from build123d import *

# Parameters (mm, degrees)
F0_W        = 76.2
F0_H        = 50.8
F2_DEPTH    = 25.4
F1_W        = 76.2
F1_H        = 8.89
F3_DEPTH    = 8.89
F4_R        = 2.54
F6_DEPTH    = 16.51
F7_R        = 5.08
F8_T        = 2.54
F8_T3_DEPTH = 10.16
F8_T5_DEPTH = 37.1348
F8_T7_DEPTH = 37.1348
F8_T9_DEPTH = 81.28


# Not quite as in the source:
# - a shell that OpenCascade refuses in one call is made with other operations: the cavity is built on its own and cut out


with BuildPart() as f2:
    # F0 (on Top) → F2 (new body)
    with BuildSketch(Plane.XY):
        Rectangle(F0_W, F0_H)
    extrude(amount=F2_DEPTH)

    # F1 (on face) → F3 (cut)
    with BuildSketch(Plane.XY):
        with Locations((0, -10.795)):
            Rectangle(F1_W, F1_H)
    extrude(amount=F3_DEPTH, mode=Mode.SUBTRACT)

    # F4
    f4_edges = [f2.edges().sort_by_distance(p)[0] for p in [
        (-38.1, 9.525, 0),
        (0, 25.4, 0),
        (38.1, 9.525, 0),
        (-38.1, -20.32, 0),
        (0, -25.4, 0),
        (38.1, -20.32, 0),
        (-38.1, 25.4, 12.7),
        (-38.1, -25.4, 12.7),
        (38.1, -25.4, 12.7),
        (38.1, 25.4, 12.7),
    ]]
    fillet(f4_edges, radius=F4_R)

    # F5 (on face) → F6 (cut, through all)
    with BuildSketch(Plane.XY.offset(25.4)):
        Polygon((6.0452, 25.4), (-6.0452, 25.4), (-6.0452, -6.35), (-6.0452, -8.89), (6.0452, -8.89), (6.0452, -6.35), align=None)
        with BuildLine():
            Line((6.0452, -8.89), (-6.0452, -8.89))
            ThreePointArc((-6.0452, -8.89), (0, -14.9352), (6.0452, -8.89))
        make_face()
    extrude(amount=-F6_DEPTH, mode=Mode.SUBTRACT)

    # F7
    f7_edges = [f2.edges().sort_by_distance(p)[0] for p in [
        (-6.0452, 9.525, 8.89),
        (6.0452, 9.525, 8.89),
    ]]
    fillet(f7_edges, radius=F7_R)

    # F8: shell of thickness 2.54, made by hand


with BuildPart() as f8_core1:
    # F8_t2: copy of F2
    add(f2.part)

    # the walls: a layer under each face that stays
    f8_faces = [f8_core1.faces().sort_by_distance(p)[0] for p in [
        (23.7066666667, 25.4, 21.59),
        (-6.0452, 8.255, 17.145),
        (-4.5573024484, 9.525, 10.3778975516),
        (0, 9.525, 8.89),
        (4.5573024484, 9.525, 10.3778975516),
        (6.0452, 8.255, 17.145),
        (0, -6.35, 6.985),
        (0, -14.9352, 17.145),
        (-25.4, -13.7583333333, 8.89),
        (38.1, 0, 13.97),
        (0, -25.4, 13.97),
        (-38.1, 0, 13.97),
        (0, 8.255, 0),
        (0, -15.24, 4.445),
        (0, -19.05, 0),
    ]]
    thicken(f8_faces, amount=-F8_T, mode=Mode.SUBTRACT)

    # F8_s4 → F8_t3 (cut)
    with BuildSketch(Plane.XY.offset(6.35)):
        Polygon((-6.0198, -6.3754), (-8.5852, -6.35), (-8.5852, -3.81), (-6.0452, -3.81), align=None)
        Polygon((6.0198, -6.3754), (8.5852, -6.35), (8.5852, -3.81), (6.0452, -3.81), align=None)
    extrude(amount=F8_T3_DEPTH, mode=Mode.SUBTRACT)

    # F8_s6 → F8_t5 (cut)
    with BuildSketch(Plane.YZ.offset(3.5052)):
        Polygon((-6.3754, 8.8646), (-3.81, 8.89), (-3.81, 11.43), (-6.35, 11.43), align=None)
    extrude(amount=F8_T5_DEPTH, mode=Mode.SUBTRACT)

    # F8_s8 → F8_t7 (cut)
    with BuildSketch(Plane.YZ.offset(-40.64)):
        Polygon((-6.3754, 8.8646), (-3.81, 8.89), (-3.81, 11.43), (-6.35, 11.43), align=None)
    extrude(amount=F8_T7_DEPTH, mode=Mode.SUBTRACT)

    # F8_s10 → F8_t9 (cut)
    with BuildSketch(Plane.YZ.offset(-40.64)):
        Polygon((-15.2146, 8.8646), (-15.24, 11.43), (-17.78, 11.43), (-17.78, 8.89), align=None)
    extrude(amount=F8_T9_DEPTH, mode=Mode.SUBTRACT)


with BuildPart() as f2_1:
    add(f2.part)

    # what is left inside the walls is the cavity
    f8_cavity = [f8_core1.part.solids().sort_by_distance(p)[0] for p in [
        (-17.78, 7.62, 25.3746),
    ]]
    add(f8_cavity, mode=Mode.SUBTRACT)


solid = f2_1.part
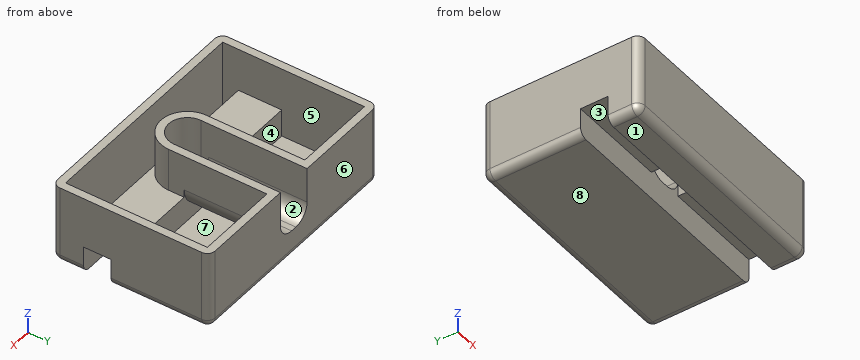
Check sheet for the modelled part. Datum: model origin and axes. Units: mm. Face numbers are marked on the shaded views. A direction names the side the tool comes from. Round coordinates to 2 decimals unless told otherwise and drop trailing zeros. Loops run counter-clockwise (first coordinate to the right, second up) from the corner with the lowest first, then second, coordinate; pieces in that order, holes last.
1. Set-up check for the marked faces 1, 2, 3, 4 and 5: record each of +Z, -Z, +X, -X, +Y, -Y from which the full face is reachable in a straight line by a thin tool's end or side.
2. Scan lines: probe 1 along X at (y, z) = (-8, 15.5); probe 2 along Y at (x, z) = (-25.5, 11.25); probe 3 along Y at (x, z) = (-19.5, 5.5). Record each from-to range of solid material in increasing order.
3. Mould release check, pull along Y, two halves, no side actions. Record for the marked faces 6, 7 and 8: released by +Y, released by -Y, zero draft, split by the parting line, or undercut.
4. Gauge pin test, flat ends, axial feed: pin 1 Ø1 at (x, z) = (-3.5, 17.5) entering from +Y; pin 2 Ø5 at (x, y) = (28.5, 15) entering from +Z; pin 3 Ø1 at (x, y) = (0, 6.5) entering from +Z. Record the tip position at first contact, or that the pin passes through.
5. Sectioned sample at C-C on y = 4. Record the boundary of the cut face in (x, z).
6. Sectioned sample at D-D on z = 18.5. Record the boundary of the cut face in (x, y).
7. Sectioned sample at A-A on x = 0. Record the boundary of the cut face in (y, z), and give its area (3 significant figures).
8. Sectioned sample at B-B on z = 5. Record the boundary of the cut face in (x, y), and give its area (3 significant figures).
Recorded:
1. face 1: -Z, +X, -X, +Y, -Y
1. face 2: +Z, +Y
1. face 3: -Z, +X, -X
1. face 4: none
1. face 5: +Z
2. probe 1: x = -38.1 to -35.56, -8.59 to -6.05, 6.05 to 8.59, 35.56 to 38.1
2. probe 2: y = -25.4 to -22.86, -17.78 to -3.81, 22.86 to 25.4
2. probe 3: y = -25.4 to -22.86, -17.78 to -15.24, -6.35 to -3.81, 22.86 to 25.4
3. face 6: released by +Y
3. face 7: undercut
3. face 8: zero draft
4. pin 1: stops at y = -13.42
4. pin 2: stops at z = 2.54
4. pin 3: stops at z = 8.89
5. outline: (-38.1, 2.54) arc R2.54 ccw to (-35.56, 0) - (35.56, 0) arc R2.54 ccw to (38.1, 2.54) - (38.1, 25.4) - (35.56, 25.4) - (35.56, 2.54) - (-35.56, 2.54) - (-35.56, 25.4) - (-38.1, 25.4) - close; (-8.59, 13.97) arc R7.62 ccw to (-0.97, 6.35) - (0.97, 6.35) arc R7.62 ccw to (8.59, 13.97) - (8.59, 25.4) - (6.05, 25.4) - (6.05, 13.97) arc R5.08 cw to (0.97, 8.89) - (-0.97, 8.89) arc R5.08 cw to (-6.05, 13.97) - (-6.05, 25.4) - (-8.59, 25.4) - close
6. outline: (-38.1, -22.86) arc R2.54 ccw to (-35.56, -25.4) - (35.56, -25.4) arc R2.54 ccw to (38.1, -22.86) - (38.1, 22.86) arc R2.54 ccw to (35.56, 25.4) - (6.05, 25.4) - (6.05, -8.89) arc R6.05 cw to (-6.05, -8.89) - (-6.05, 25.4) - (-35.56, 25.4) arc R2.54 ccw to (-38.1, 22.86) - close; hole (-35.56, -22.86) - (35.56, -22.86) - (35.56, 22.86) - (8.59, 22.86) - (8.59, -8.89) arc R8.59 cw to (-8.59, -8.89) - (-8.59, 22.86) - (-35.56, 22.86) - close
7. outline: (-25.4, 2.54) arc R2.54 ccw to (-22.86, 0) - (-15.24, 0) - (-15.24, 8.89) - (-14.94, 8.89) - (-14.94, 25.4) - (-17.48, 25.4) - (-17.48, 11.43) - (-17.78, 11.43) - (-17.78, 2.54) - (-22.86, 2.54) - (-22.86, 25.4) - (-25.4, 25.4) - close; (-6.35, 0) - (22.86, 0) arc R2.54 ccw to (25.4, 2.54) - (25.4, 8.89) - (-6.35, 8.89) - close; hole (-3.81, 2.54) - (22.86, 2.54) - (22.86, 6.35) - (-3.81, 6.35) - close
7. area: 321 mm2
8. outline: (-38.1, -22.86) arc R2.54 ccw to (-35.56, -25.4) - (35.56, -25.4) arc R2.54 ccw to (38.1, -22.86) - (38.1, -15.24) - (-38.1, -15.24) - close; (-38.1, -6.35) - (38.1, -6.35) - (38.1, 22.86) arc R2.54 ccw to (35.56, 25.4) - (-35.56, 25.4) arc R2.54 ccw to (-38.1, 22.86) - close; hole (-35.56, -22.86) - (35.56, -22.86) - (35.56, -17.78) - (-35.56, -17.78) - close; hole (-35.56, -3.81) - (35.56, -3.81) - (35.56, 22.86) - (-35.56, 22.86) - close
8. area: 930 mm2
